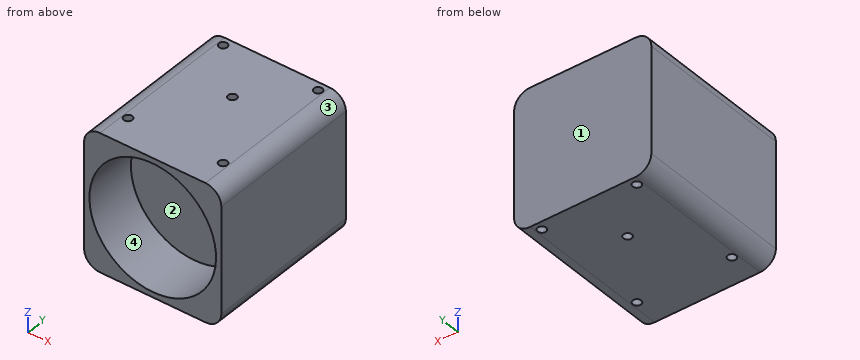
```python
from build123d import *

# Parameters (mm, degrees)
SKETCH1_W                  = 26
SKETCH1_H                  = 26
BOSS_EXTRUDE1_DEPTH        = 15
FILLET1_R                  = 3
SKETCH2_R                  = 12
CUT_EXTRUDE1_DEPTH         = 10
M2_TAPPED_HOLE2_AT_2_COUNT = 2
M2_TAPPED_HOLE2_AT_2_PITCH = 18
M2_TAPPED_HOLE2_AT_3_COUNT = 2
M2_TAPPED_HOLE2_AT_3_PITCH = 12.870120435
M2_TAPPED_HOLE2_AT_4_COUNT = 2
M2_TAPPED_HOLE2_AT_4_PITCH = 22.9
M2_TAPPED_HOLE2_AT_5_COUNT = 2
M2_TAPPED_HOLE2_AT_5_PITCH = 29.127478435


with BuildPart() as part:
    # Sketch1 → Boss-Extrude1 (new, symmetric)
    with BuildSketch(Plane(origin=(0, 0, 0), x_dir=(1, 0, 0), z_dir=(0, 1, 0))):
        Rectangle(SKETCH1_W, SKETCH1_H)
    extrude(amount=BOSS_EXTRUDE1_DEPTH, both=True)

    # Fillet1
    fillet1_edges = [part.edges().sort_by_distance(p)[0] for p in [
        (13, 0, 13),
        (-13, 0, 13),
        (-13, 0, -13),
        (13, 0, -13),
    ]]
    fillet(fillet1_edges, radius=FILLET1_R)

    # Sketch2 → Cut-Extrude1 (cut)
    with BuildSketch(Plane.XZ.offset(15)):
        with Locations(Location((0, 0, 0), (0, 0, 270))):
            Circle(SKETCH2_R)
    extrude(amount=-CUT_EXTRUDE1_DEPTH, mode=Mode.SUBTRACT)

    # Sketch4 → M2 Tapped Hole2 (revolve, cut)
    with BuildSketch(Plane(origin=(-9, 13.4, 13), x_dir=(0, -1, 0), z_dir=(1, 0, 0))):
        Polygon((0, 0), (0, 2.980688495), (0.8, 2.5), (0.8, 0), align=None)
    m2_tapped_hole2 = revolve(axis=Axis((-9, 13.4, 19.35), (0, 0, -1)), mode=Mode.SUBTRACT)

    # M2 Tapped Hole2 at 2: M2 Tapped Hole2 ×2
    with Locations(*[(i * M2_TAPPED_HOLE2_AT_2_PITCH, 0, 0) for i in range(1, M2_TAPPED_HOLE2_AT_2_COUNT)]):
        add(m2_tapped_hole2, mode=Mode.SUBTRACT)

    # M2 Tapped Hole2 at 3: M2 Tapped Hole2 ×2
    with Locations(*[Vector(0.6992941554637311, -0.7148340255851474, 0) * (i * M2_TAPPED_HOLE2_AT_3_PITCH) for i in range(1, M2_TAPPED_HOLE2_AT_3_COUNT)]):
        add(m2_tapped_hole2, mode=Mode.SUBTRACT)

    # M2 Tapped Hole2 at 4: M2 Tapped Hole2 ×2
    with Locations(*[(0, -i * M2_TAPPED_HOLE2_AT_4_PITCH, 0) for i in range(1, M2_TAPPED_HOLE2_AT_4_COUNT)]):
        add(m2_tapped_hole2, mode=Mode.SUBTRACT)

    # M2 Tapped Hole2 at 5: M2 Tapped Hole2 ×2
    with Locations(*[Vector(0.6179731637247914, -0.7861991916276512, 0) * (i * M2_TAPPED_HOLE2_AT_5_PITCH) for i in range(1, M2_TAPPED_HOLE2_AT_5_COUNT)]):
        add(m2_tapped_hole2, mode=Mode.SUBTRACT)

    # Mirror1: M2 Tapped Hole2 across plane
    add(m2_tapped_hole2.mirror(Plane.XY), mode=Mode.SUBTRACT)

    # Mirror1 copy 1 sketch → Mirror1 copy 1 (revolve, cut)
    with BuildSketch(Plane(origin=(9, 13.4, -13), x_dir=(0, -1, 0), z_dir=(1, 0, 0))):
        Polygon((0, 0), (0, -2.980688495), (0.8, -2.5), (0.8, 0), align=None)
    revolve(axis=Axis((9, 13.4, -19.35), (0, 0, -1)), mode=Mode.SUBTRACT)

    # Mirror1 copy 2 sketch → Mirror1 copy 2 (revolve, cut)
    with BuildSketch(Plane(origin=(0, 4.2, -13), x_dir=(0, -1, 0), z_dir=(1, 0, 0))):
        Polygon((0, 0), (0, -2.980688495), (0.8, -2.5), (0.8, 0), align=None)
    revolve(axis=Axis((0, 4.2, -19.35), (0, 0, -1)), mode=Mode.SUBTRACT)

    # Mirror1 copy 3 sketch → Mirror1 copy 3 (revolve, cut)
    with BuildSketch(Plane(origin=(-9, -9.5, -13), x_dir=(0, -1, 0), z_dir=(1, 0, 0))):
        Polygon((0, 0), (0, -2.980688495), (0.8, -2.5), (0.8, 0), align=None)
    revolve(axis=Axis((-9, -9.5, -19.35), (0, 0, -1)), mode=Mode.SUBTRACT)

    # Mirror1 copy 4 sketch → Mirror1 copy 4 (revolve, cut)
    with BuildSketch(Plane(origin=(9, -9.5, -13), x_dir=(0, -1, 0), z_dir=(1, 0, 0))):
        Polygon((0, 0), (0, -2.980688495), (0.8, -2.5), (0.8, 0), align=None)
    revolve(axis=Axis((9, -9.5, -19.35), (0, 0, -1)), mode=Mode.SUBTRACT)


solid = part.part
```
The model under review builds one solid part; all positions refer to its coordinate system, in mm. Face numbers are marked on the shaded views. Round coordinates to 2 decimals unless told otherwise and drop trailing zeros. Order: outer loops, then holes, each group sorted by start corner. A loop starts at its lowest first (then second) coordinate and runs counter-clockwise, first axis right, second up. Notation, with made-up numbers: (-36.5, -32) -> (-14.5, -32) arc R9 cw to (-14.5, -28) -> close; hole circle Ø8 at (-5, 49.5). An arc over 180 degrees is marked (long way). Use a Markdown table: item, result.
Q1. Mouldability with a two-part tool opening along X and no side actions: class the marked faces 1, 2, 3 and 4 as +X half, -X half, draft (parallel to the pull), parting line (faces both ways), or undercut.
Values:
| item | result |
|---|---|
| face 1 | draft |
| face 2 | undercut |
| face 3 | +X half |
| face 4 | undercut |
Q2. We need section C-C on x = 1.25. Write out the cut boundary in (y, z).
Values:
| item | result |
|---|---|
| outline | (-15, -13) -> (15, -13) -> (15, 13) -> (-15, 13) -> (-15, 11.93) -> (-5, 11.93) -> (-5, -11.93) -> (-15, -11.93) -> close |
Q3. We need section B-B on z = 0. Write out the cut boundary in (x, y), then the cut area to 3 significant figures.
Values:
| item | result |
|---|---|
| outline | (-13, -15) -> (-12, -15) -> (-12, -5) -> (12, -5) -> (12, -15) -> (13, -15) -> (13, 15) -> (-13, 15) -> close |
| area | 540 mm^2 |
Q4. We need section A-A on y = -7. Write out the cut boundary in (x, z).
Values:
| item | result |
|---|---|
| outline | (-13, -10) arc R3 ccw to (-10, -13) -> (10, -13) arc R3 ccw to (13, -10) -> (13, 10) arc R3 ccw to (10, 13) -> (-10, 13) arc R3 ccw to (-13, 10) -> close; hole circle Ø24 at (0, 0) |
Q5. For line 1 (Y direction, x = -9, z = 11.1); line 2 (X direction, y = -7.75, z = 0); line 3 (Y direction, x = -5.5, z = 5.5), list the stretches that pass through material, from the lowest coordinate up.
Values:
| item | result |
|---|---|
| line 1 | y = -15 to -10.3, -8.7 to 12.6, 14.2 to 15 |
| line 2 | x = -13 to -12, 12 to 13 |
| line 3 | y = -5 to 15 |
Q6. Clearance check with flat-ended pins moving along their axes: P1, Ø14.5, axis at x = 0, z = 0, coming from the -Y side; P2, Ø1.3, axis at x = 9, y = -9.5, coming from the +Z side; P3, Ø1.3, axis at x = 9, y = 13.4, coming from the -Z side. State where each tip first meets the part, or that it passes through.
Values:
| item | result |
|---|---|
| P1 | stops at y = -5 |
| P2 | stops at z = 10.41 |
| P3 | stops at z = -10.41 |
